```python
from build123d import *

# Parameters (mm, degrees)
BOSS_EXTRUDE1_DEPTH = 10
SKETCH3_R           = 3.8
CUT_EXTRUDE1_DEPTH  = 46.041452221


with BuildPart() as part:
    # Sketch1 → Boss-Extrude1 (new body)
    with BuildSketch(Plane(origin=(0, 0, 0), x_dir=(1, 0, 0), z_dir=(0, 1, 0))):
        Polygon((-11.5, -6.639528096), (-11.5, 6.639528096), (-14.5, 6.639528096), (-14.5, -6.639528096), (-10.25, -11.068500464), (-10.25, -36.279056191), (-5.25, -36.279056191), (-5.25, -16.279056191), (5.25, -16.279056191), (5.25, -36.279056191), (10.25, -36.279056191), (10.25, -11.068500464), (14.5, -6.639528096), (14.5, 6.639528096), (11.5, 6.639528096), (11.5, -6.639528096), (0, -13.279056191), align=None)
    extrude(amount=BOSS_EXTRUDE1_DEPTH)

    # Sketch3 → Cut-Extrude1 (cut, through all)
    with BuildSketch(Plane.ZY.offset(10.25)):
        with Locations((19.079056191, 5)):
            Circle(SKETCH3_R)
        with Locations((29.079056191, 5)):
            Circle(SKETCH3_R)
    extrude(amount=-CUT_EXTRUDE1_DEPTH, mode=Mode.SUBTRACT)


solid = part.part
```
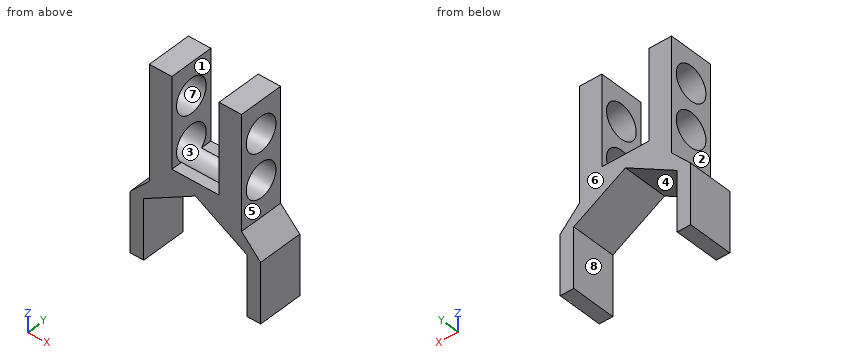
The listing builds one solid part. Answer for the finished solid, in the listing's coordinates (mm). Face numbers are marked on the shaded views. A direction names the side the tool comes from. Coordinates: 2 decimals unless noted, no trailing zeros. Write each loop counter-clockwise with the first axis right and the second up, starting at its lowest first coordinate (ties: lowest second). Pieces come first, ordered by that corner, then holes. Notation, with made-up numbers: (59, 83.5) - (89, 83.5) arc R23 ccw to (89, 103.5) - close; hole circle Ø8 at (36.5, 33.25). An arc over 180 degrees is marked (long way). One line per item, written item: value.
1) Find section A-A (z = 4). Give the vertices of the cut face in (x, y), and give its area (3 significant figures).
Geometry check:
outline: (-14.5, 0) - (-11.5, 0) - (-11.5, 10) - (-14.5, 10) - close; (11.5, 0) - (14.5, 0) - (14.5, 10) - (11.5, 10) - close
area: 60.0 mm2
2) Find section C-C (y = 9.25). Give the vertices of the cut face in (x, z).
Geometry check:
outline: (-14.5, -6.64) - (-11.5, -6.64) - (-11.5, 6.64) - (0, 13.28) - (11.5, 6.64) - (11.5, -6.64) - (14.5, -6.64) - (14.5, 6.64) - (10.25, 11.07) - (10.25, 36.28) - (5.25, 36.28) - (5.25, 16.28) - (-5.25, 16.28) - (-5.25, 36.28) - (-10.25, 36.28) - (-10.25, 11.07) - (-14.5, 6.64) - close
3) Each of these flat-tipped pins is pushed along its axis until it touches: pin 1 Ø0.7 at (x, y) = (-1, 8.5) entering from +Z; pin 2 Ø6 at (y, z) = (8.5, 15.5) entering from +X; pin 3 Ø2 at (x, z) = (-11, 21) entering from +Y; pin 4 Ø5 at (x, y) = (-8.5, 5.5) entering from -Z. Where does it stop, or does it pass through?
Geometry check:
pin 1: stops at z = 16.28
pin 2: stops at x = 10.25
pin 3: stops at y = 10
pin 4: stops at z = 6.93
4) Find section D-D (x = 2.5). Give the vertices of the cut face in (y, z).
Geometry check:
outline: (0, 11.84) - (10, 11.84) - (10, 16.28) - (7.57, 16.28) arc R3.8 cw to (2.43, 16.28) - (0, 16.28) - close
5) Find section B-B (y = 5). Count the separate pieces of the cut face and the enclosed holes in it, and give its area (3 significant figures).
Geometry check:
separate pieces: 5
enclosed holes: 0
area: 257 mm2
6) A tool of negligible diameter and unlimited length cuts with its end or side. For the marked faces 1, 2, 3, 4 and 5, from which of +Z, -Z, +X, -X, +Y, -Y can it reach the whole face along a straight path? Write none if from no direction.
Geometry check:
face 1: +Z, +Y, -Y
face 2: +Z, -X, +Y, -Y
face 3: +X, -X
face 4: -Z, +Y, -Y
face 5: +Z, +X, +Y, -Y
7) Consider line 1 along X through (y, z) = (8.5, 4.5); line 2 along X through (y, z) = (8.75, 24.5); line 3 along Z through (x, y) = (-6.5, 3.25). Determine where each line is inside the solid, lowest interval first. Write a range as from..to.
Geometry check:
line 1: x = -14.5..-11.5, 11.5..14.5
line 2: x = -10.25..-5.25, 5.25..10.25
line 3: z = 9.53..15.71, 22.45..25.71, 32.45..36.28
8) For a pull along Y with two mould halves and no side action, classify the marked faces 6, 7 and 8 as pulls with the +Y half, pulls with the -Y half, needs draft (parallel to the pull), parting line crosses it, or undercut.
Geometry check:
face 6: pulls with the +Y half
face 7: undercut
face 8: needs draft
